Autodesk Inventor part; units mm, degrees
ref_plane "YZ Plane" through (0, 0, 0) normal (1, 0, 0) x (0, 1, 0)
ref_plane "XZ Plane" through (0, 0, 0) normal (0, 1, 0) x (-1, 0, 0)
ref_plane "XY Plane" through (0, 0, 0) normal (0, 0, 1) x (1, 0, 0)
sketch "Sketch1" plane through (0, 0, 0) normal (0, 0, 1) x (1, 0, 0)
  circle A0 centre (0, 0) radius 1.75
  circle A1 centre (0, 0) radius 1.85
  circle A2 centre (0, 0) radius 3.85
  point P0 (0, 0)
  dimension "d0" = 0.1
  dimension "d1" = 2
extrude "Extrusion1" add sketch "Sketch1" against normal blind 5 contours A2
sketch "Sketch2" plane through (0, 0, 0) normal (0, 0, 1) x (1, 0, 0)
  point P0 (0, 0)
sketch "Sketch3" plane through (0, 0, 0) normal (0, 0, 1) x (1, 0, 0)
  circle A0 centre (0, 0) radius 3.85
extrude "Extrusion2" add sketch "Sketch3" along normal blind 24
sketch "Sketch4" plane through (0, 0, 24) normal (0, 0, 1) x (1, 0, 0)
  line L0 (12.065, -6.985) -> (-12.065, -6.985)
  line L1 (-12.065, -6.985) -> (-12.065, 6.985)
  line L2 (-12.065, 6.985) -> (12.065, 6.985)
  line L3 (12.065, 6.985) -> (12.065, -6.985)
  circle A0 centre (0, 0) radius 1.85
  line L4 (12.065, -6.985) -> (-12.065, 6.985) construction
  line L5 (-12.065, -6.985) -> (12.065, 6.985) construction
  line L6 (12.065, 12.065) -> (-12.065, 12.065) construction
  line L7 (-12.065, 12.065) -> (-12.065, 26.035) construction
  line L8 (-12.065, 26.035) -> (12.065, 26.035) construction
  line L9 (12.065, 26.035) -> (12.065, 12.065) construction
  line L10 (12.065, 12.065) -> (-12.065, 26.035) construction
  line L11 (-12.065, 12.065) -> (12.065, 26.035) construction
  line L12 (12.065, -8.89) -> (-16.51, -8.89)
  line L13 (-16.51, -8.89) -> (-16.51, 8.89)
  line L14 (-16.51, 8.89) -> (12.065, 8.89)
  line L15 (16.51, -8.89) -> (-16.51, 8.89) construction
  line L16 (-16.51, -8.89) -> (12.065, 6.4965) construction
  line L17 (12.065, -8.89) -> (12.065, 8.89)
  point P0 (0, 0)
  point P1 (0, 19.05)
  dimension "d6" = 24.13
  dimension "d7" = 13.97
  dimension "d10" = 19.05
  dimension "d16" = 17.78
extrude "Extrusion3" add sketch "Sketch4" along normal blind 1.5 contours L17 L12 L13 L14 L2 L1 L0 | L0 L1 L2 L3 | A0
extrude "Extrusion4" add sketch "Sketch4" along normal blind 6 contours L0 L1 L2 L3 | A0
fillet "Fillet1" radius 3.175 8 edges at (-12.065, 6.985, 27.75) (12.065, 6.985, 27.75) (12.065, -6.985, 27.75) (-12.065, -6.985, 27.75) (-16.51, -8.89, 24.75) (12.065, 8.89, 24.75) (-16.51, 8.89, 24.75) (12.065, -8.89, 24.75)
properties part number "Button Cover"
Read the model definition and answer for the solid it produces. Units are mm, in the model's axes. A direction names the side the tool comes from. Round coordinates to 2 decimals unless told otherwise and drop trailing zeros. Write each loop counter-clockwise with the first axis right and the second up, starting at its lowest first coordinate (ties: lowest second). Pieces come first, ordered by that corner, then holes. Notation, with made-up numbers: (-29, 25) - (7, 25) arc R22 ccw to (7, 41) - close; hole circle Ø4 at (42.25, 84.5). An arc over 180 degrees is marked (long way). Use a Markdown table: item, result.
(1) Which of the six approach directions +Z, -Z, +X, -X, +Y, -Y give full straight-line access (tool end or side, diameter ignored) to faces 4 (the cylindrical face through (11.11, -6.08, 27.78)), 5 (the flat face through (0, -6.985, 28)), 6 (the flat face through (0, 6.985, 28))?
Reported:
| item | result |
|---|---|
| face 4 | +Z, +X, -Y |
| face 5 | +Z, +X, -X, -Y |
| face 6 | +Z, +X, -X, +Y |
(2) The part is cut by section C-C (z = 9). Write down the section's boundary in (x, y).
Reported:
| item | result |
|---|---|
| outline | circle Ø7.7 at (0, 0) |
(3) The mould has two halves that part along X. Classify faces 1 (the flat face through (-6, 0, 24)), 2 (the flat face through (0, 0, 0)), 3 (the cylindrical face through (-0.83, -3.76, 9.7)): released by +X, released by -X, zero draft, split by the parting line, or undercut.
Reported:
| item | result |
|---|---|
| face 1 | zero draft |
| face 2 | undercut |
| face 3 | split by the parting line |
(4) The part is cut by section B-B (x = 6.5). Write down the section's boundary in (y, z) (3 decimals).
Reported:
| item | result |
|---|---|
| outline | (-8.89, 24) - (8.89, 24) - (8.89, 25.5) - (6.985, 25.5) - (6.985, 30) - (-6.985, 30) - (-6.985, 25.5) - (-8.89, 25.5) - close |
(5) The part is cut by section D-D (x = -9.75). Write down the section's boundary in (y, z).
Reported:
| item | result |
|---|---|
| outline | (-8.89, 24) - (8.89, 24) - (8.89, 25.5) - (6.87, 25.5) - (6.87, 30) - (-6.87, 30) - (-6.87, 25.5) - (-8.89, 25.5) - close |
(6) Each of these flat-tipped pins is pushed along its axis until it touches: pin 1 Ø2 at (x, z) = (4, 11) entering from -Y; pin 2 Ø3.5 at (x, z) = (-4.5, 28) entering from -Y (3 decimals); pin 3 Ø8 at (x, y) = (-9.5, 4) entering from -Z. Where does it stop, or does it pass through?
Reported:
| item | result |
|---|---|
| pin 1 | y = -2.41 |
| pin 2 | y = -6.985 |
| pin 3 | z = 24 |
(7) The part is cut by section A-A (y = 0). Write down the section's boundary in (x, z) (3 decimals).
Reported:
| item | result |
|---|---|
| outline | (-16.51, 24) - (-3.85, 24) - (-3.85, -5) - (-1.85, -5) - (-1.85, 0) - (1.85, 0) - (1.85, -5) - (3.85, -5) - (3.85, 24) - (12.065, 24) - (12.065, 30) - (-12.065, 30) - (-12.065, 25.5) - (-16.51, 25.5) - close |
(8) Straight lines are drawn through the part: line 1 along Y through (x, z) = (0, -3.7); line 2 along Z through (x, y) = (6, -5.75); line 3 along Z through (x, y) = (-2.5, 7.25). For each, find the intervals that lie inside material, in ascending order. Write a range as [from, to].
Reported:
| item | result |
|---|---|
| line 1 | [-3.85, -1.85], [1.85, 3.85] |
| line 2 | [24, 30] |
| line 3 | [24, 25.5] |
